Here's how the part is built. I have some questions about the finished solid (model axes, mm). Face numbers are marked on the shaded views. A direction names the side the tool comes from. Round coordinates to 2 decimals unless told otherwise and drop trailing zeros. Loops run counter-clockwise (first coordinate to the right, second up) from the corner with the lowest first, then second, coordinate; pieces in that order, holes last. Notation, with made-up numbers: M 0,32 L 43,32 A4 ccw 43,36 Z; hole C -2,61.5 d3. An arc over 180 degrees is marked long. Answer as CSV lines item,"result".
```python
from build123d import *

# Parameters (mm, degrees)
SKETCH1_R          = 50
SKETCH1_R_2        = 38.75
EXTRUDE1_DEPTH     = 10
CUT_EXTRUDE1_DEPTH = 11
CIRPATTERN1_COUNT  = 4


with BuildPart() as part:
    # Sketch1 → Extrude1 (new body)
    with BuildSketch(Plane.XY):
        Circle(SKETCH1_R)
        Circle(SKETCH1_R_2, mode=Mode.SUBTRACT)
    extrude(amount=EXTRUDE1_DEPTH)

    # Sketch2 → Cut-Extrude1 (cut, through all)
    with BuildSketch(Plane.XY.offset(10)):
        with BuildLine():
            Line((31.25170097, 39.029875563), (28.425692604, 36.203867197))
            Line((28.425692604, 36.203867197), (36.203867197, 28.425692604))
            Line((36.203867197, 28.425692604), (39.029875563, 31.25170097))
            ThreePointArc((39.029875563, 31.25170097), (35.355339059, 35.355339059), (31.25170097, 39.029875563))
        make_face()
    cut_extrude1 = extrude(amount=-CUT_EXTRUDE1_DEPTH, mode=Mode.SUBTRACT)

    # CirPattern1: Cut-Extrude1 ×4 about axis
    cirpattern1_axis = Axis((0, 0, 0), (0, 0, 1))
    for i in range(1, CIRPATTERN1_COUNT):
        add(cut_extrude1.rotate(cirpattern1_axis, i * 360 / CIRPATTERN1_COUNT), mode=Mode.SUBTRACT)

    # Sketch3 → Cut-Revolve1 (revolve, cut)
    with BuildSketch(Plane(origin=(0, 0, 0), x_dir=(1, 0, 0), z_dir=(0, 1, 0))):
        Polygon((50, 0), (45.5, 0), (50, -2.922334169), align=None)
    revolve(axis=Axis((0, 0, 0), (0, 0, -1)), mode=Mode.SUBTRACT)


solid = part.part
```
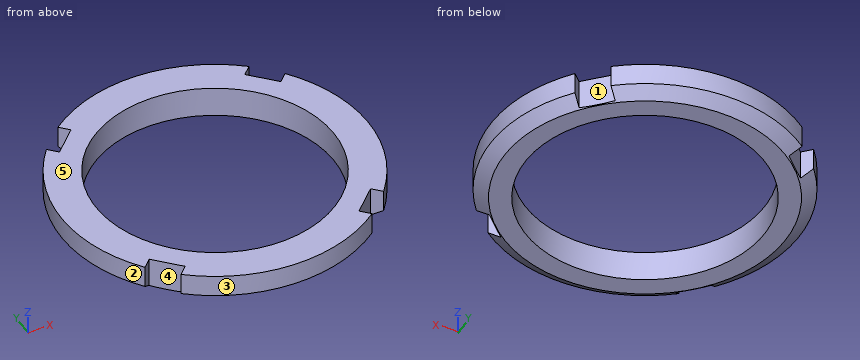
1. Which directions (+Z, -Z, +X, -X, +Y, -Y) give clear straight access to the entire face, cutting with the end or side of a thin tool? Please do the marked faces 4 and 5.
Evaluation:
face 4,"+Z, -Z"
face 5,"+Z, +X, -X, +Y, -Y"
2. For P1, Ø1.5, axis at x = 16, z = 9, coming from the -Y side; P2, Ø1, axis at x = -13, z = 5.5, coming from the +Y side; P3, Ø4, axis at x = 11, z = 1.5, coming from the +Y side, each with a flat end and sliding along its axis, tell me the tip position at first contact or that it passes through.
Evaluation:
P1,"stops at y = -47.62"
P2,"stops at y = 48.41"
P3,"stops at y = 49.07"
3. We'd pull the mould along X, two halves only. Please class the marked faces 1, 2 and 3: pulls with the +X half, pulls with the -X half, needs draft (parallel to the pull), parting line crosses it, or undercut.
Evaluation:
face 1,"undercut"
face 2,"pulls with the -X half"
face 3,"parting line crosses it"
4. I want a section at A-A, the plane y = 0. Please give me the cut outline in (x, z), and give its area (3 significant figures).
Evaluation:
outline,"M -50,2.92 L -45.5,0 L -38.75,0 L -38.75,10 L -50,10 Z; M 38.75,0 L 45.5,0 L 50,2.92 L 50,10 L 38.75,10 Z"
area,"212 mm²"
5. If I drill on line 1 (Y direction, x = 8, z = 4.75); line 2 (X direction, y = 7.5, z = 1.25); line 3 (X direction, y = 36, z = 2), over which ranges is the centre line in solid material (lowest first)? Write a range as [from, to].
Evaluation:
line 1,"y = [-49.36, -37.92], [37.92, 49.36]"
line 2,"x = [-46.83, -38.02], [38.02, 46.83]"
line 3,"x = [-28.63, -14.34], [14.34, 28.63]"
6. I want a section at C-C, the plane z = 5.75. Please give me the cut outline in (x, y).
Evaluation:
outline,"M -39.03,-31.25 L -36.2,-28.43 L -28.43,-36.2 L -31.25,-39.03 A50 ccw 31.25,-39.03 L 28.43,-36.2 L 36.2,-28.43 L 39.03,-31.25 A50 ccw 39.03,31.25 L 36.2,28.43 L 28.43,36.2 L 31.25,39.03 A50 ccw -31.25,39.03 L -28.43,36.2 L -36.2,28.43 L -39.03,31.25 A50 ccw Z; hole C 0,0 d77.5"
